The model under review builds one solid part; all positions refer to its coordinate system, in mm. A direction names the side the tool comes from. Round coordinates to 2 decimals unless told otherwise and drop trailing zeros. Write each loop counter-clockwise with the first axis right and the second up, starting at its lowest first coordinate (ties: lowest second). Pieces come first, ordered by that corner, then holes. Notation, with made-up numbers: (80.5, 36.5) - (124.5, 36.5) arc R29 cw to (124.5, 75.5) - close; hole circle Ø9 at (-11.75, -21.5). An arc over 180 degrees is marked (long way). Return JSON: item names as keys, results as strings.
Autodesk Inventor part; units mm, degrees
ref_plane "YZ Plane" through (0, 0, 0) normal (1, 0, 0) x (0, 1, 0)
ref_plane "XZ Plane" through (0, 0, 0) normal (0, 1, 0) x (-1, 0, 0)
ref_plane "XY Plane" through (0, 0, 0) normal (0, 0, 1) x (1, 0, 0)
ref_plane "РабПлоскость1" through (0, 0, 3) normal (0, 0, 1) x (1, 0, 0)
sketch "Эскиз1" plane through (0, 0, 3) normal (0, 0, 1) x (1, 0, 0)
  circle A0 centre (0, 0) radius 101 construction
  circle A1 centre (0, 0) radius 135
  line L0 (0, 0) -> (0, 153.023) construction
  circle A2 centre (0, 101) radius 26.5
  line L1 (86.9741, 51.6188) -> (51.6188, 86.9741) construction
  line L2 (51.6188, 86.9741) -> (55.8614, 91.2168) construction
  line L3 (55.8614, 91.2168) -> (91.2168, 55.8614) construction
  line L4 (91.2168, 55.8614) -> (86.9741, 51.6188) construction
  line L5 (86.9741, 51.6188) -> (55.8614, 91.2168) construction
  line L6 (51.6188, 86.9741) -> (91.2168, 55.8614) construction
  line L7 (86.9741, 50.2046) -> (50.2046, 86.9741)
  line L8 (50.2046, 86.9741) -> (55.8614, 92.631)
  line L9 (55.8614, 92.631) -> (92.631, 55.8614)
  line L10 (92.631, 55.8614) -> (86.9741, 50.2046)
  line L11 (86.9741, 50.2046) -> (55.8614, 92.631) construction
  line L12 (50.2046, 86.9741) -> (92.631, 55.8614) construction
  line L13 (-86.9741, 51.6188) -> (-91.2168, 55.8614) construction
  line L14 (-86.9741, 50.2046) -> (-92.631, 55.8614)
  circle A3 centre (-101, 0) radius 26.5
  line L15 (-91.2168, 55.8614) -> (-55.8614, 91.2168) construction
  line L16 (-86.9741, 51.6188) -> (-55.8614, 91.2168) construction
  line L17 (-51.6188, 86.9741) -> (-86.9741, 51.6188) construction
  line L18 (-51.6188, 86.9741) -> (-91.2168, 55.8614) construction
  line L19 (-86.9741, 50.2046) -> (-55.8614, 92.631) construction
  line L20 (-50.2046, 86.9741) -> (-86.9741, 50.2046)
  line L21 (-50.2046, 86.9741) -> (-92.631, 55.8614) construction
  line L22 (-55.8614, 91.2168) -> (-51.6188, 86.9741) construction
  line L23 (-55.8614, 92.631) -> (-50.2046, 86.9741)
  line L24 (-92.631, 55.8614) -> (-55.8614, 92.631)
  line L25 (-51.6188, -86.9741) -> (-55.8614, -91.2168) construction
  line L26 (-50.2046, -86.9741) -> (-55.8614, -92.631)
  circle A4 centre (0, -101) radius 26.5
  line L27 (-55.8614, -91.2168) -> (-91.2168, -55.8614) construction
  line L28 (-51.6188, -86.9741) -> (-91.2168, -55.8614) construction
  line L29 (-86.9741, -51.6188) -> (-51.6188, -86.9741) construction
  line L30 (-86.9741, -51.6188) -> (-55.8614, -91.2168) construction
  line L31 (-50.2046, -86.9741) -> (-92.631, -55.8614) construction
  line L32 (-86.9741, -50.2046) -> (-50.2046, -86.9741)
  line L33 (-86.9741, -50.2046) -> (-55.8614, -92.631) construction
  line L34 (-91.2168, -55.8614) -> (-86.9741, -51.6188) construction
  line L35 (-92.631, -55.8614) -> (-86.9741, -50.2046)
  line L36 (-55.8614, -92.631) -> (-92.631, -55.8614)
  line L37 (86.9741, -51.6188) -> (91.2168, -55.8614) construction
  line L38 (86.9741, -50.2046) -> (92.631, -55.8614)
  circle A5 centre (101, 0) radius 26.5
  line L39 (91.2168, -55.8614) -> (55.8614, -91.2168) construction
  line L40 (86.9741, -51.6188) -> (55.8614, -91.2168) construction
  line L41 (51.6188, -86.9741) -> (86.9741, -51.6188) construction
  line L42 (51.6188, -86.9741) -> (91.2168, -55.8614) construction
  line L43 (86.9741, -50.2046) -> (55.8614, -92.631) construction
  line L44 (50.2046, -86.9741) -> (86.9741, -50.2046)
  line L45 (50.2046, -86.9741) -> (92.631, -55.8614) construction
  line L46 (55.8614, -91.2168) -> (51.6188, -86.9741) construction
  line L47 (55.8614, -92.631) -> (50.2046, -86.9741)
  line L48 (92.631, -55.8614) -> (55.8614, -92.631)
  circle A6 centre (0, 0) radius 67
  point P0 (71.4178, 71.4178)
  point P1 (-71.4178, 71.4178)
  point P2 (-71.4178, -71.4178)
  point P3 (71.4178, -71.4178)
  dimension "d0" = 202
  dimension "d1" = 53
  dimension "d2" = 1
  dimension "d3" = 1
  dimension "d6" = 360
  dimension "d8" = 34
  dimension "d9" = 34
extrude "Выдавливание1" add sketch "Эскиз1" along normal blind 3
equation "\"d9\" = d8"
properties part number "Диск_базирующий_В5" material "По умолчанию1"
(1) Add section A-A (x = 0). Write out the cut boundary in (y, z), plus the area to 3 significant figures.
Filled in:
{"outline": "(-135, 3) - (-127.5, 3) - (-127.5, 6) - (-135, 6) - close; (-74.5, 3) - (-67, 3) - (-67, 6) - (-74.5, 6) - close; (67, 3) - (74.5, 3) - (74.5, 6) - (67, 6) - close; (127.5, 3) - (135, 3) - (135, 6) - (127.5, 6) - close", "area": "90.0 mm2"}
(2) Add section C-C (z = 3.6). Give the number of separate pieces and of enclosed holes in the cut face, plus the area to 3 significant figures.
Filled in:
{"separate pieces": "1", "enclosed holes": "9", "area": "32,700 mm2"}
(3) Clearance check with a flat-ended pin moving along its axis: pin 1 Ø1.5 at (x, z) = (106, 5) entering from +Y. State where the tip first meets the part, or that it passes through.
Filled in:
{"pin 1": "stops at y = 84.54"}
(4) For faces 4 (the flat face through (-62, 32, 3)), 5 (the flat face through (-73.99, -74.5, 4.48)), list the 3-axis set-ups (+Z, -Z, +X, -X, +Y, -Y) from which the entire face can be reached by the end or side of a thin tool; tool diameter is ignored.
Filled in:
{"face 4": "-Z, +X, -X, +Y, -Y", "face 5": "+Z, -Z"}
(5) Add section D-D (y = 101). Write out the cut boundary in (x, z).
Filled in:
{"outline": "(-89.58, 3) - (-26.5, 3) - (-26.5, 6) - (-89.58, 6) - close; (26.5, 3) - (89.58, 3) - (89.58, 6) - (26.5, 6) - close"}
(6) Mouldability with a two-part tool opening along X and no side actions: class faces 1 (the flat face through (-62, 32, 6)), 2 (the cylindrical face through (-120.53, -17.91, 4.48)), 3 (the cylindrical face through (-107.13, 82.15, 4.48)) as released by +X, released by -X, zero draft, split by the parting line, or undercut.
Filled in:
{"face 1": "zero draft", "face 2": "undercut", "face 3": "split by the parting line"}
(7) Wall thickness on line 1 (Y direction, x = 54, z = 3.35); line 2 (Y direction, x = 77.5, z = 3.2); line 3 (X direction, y = 16, z = 4.75): over which ranges is each line inside the solid? List them lowest first.
Filled in:
{"line 1": "y = -123.73 to -90.77, -83.18 to -39.66, 39.66 to 83.18, 90.77 to 123.73", "line 2": "y = -110.54 to -70.99, -59.68 to -12.25, 12.25 to 59.68, 70.99 to 110.54", "line 3": "x = -134.05 to -122.12, -79.88 to -65.06, 65.06 to 79.88, 122.12 to 134.05"}
